Geometry check sheet. Reference: the model listing, model coordinates, mm. A direction names the side the tool comes from. Coordinates: 2 decimals unless noted, no trailing zeros. Write each loop counter-clockwise with the first axis right and the second up, starting at its lowest first coordinate (ties: lowest second). Pieces come first, ordered by that corner, then holes. Notation, with made-up numbers: (44.25, -11) -> (101.25, -11) arc R21 ccw to (101.25, 21) -> close; hole circle Ø2 at (-17.75, -11.75). An arc over 180 degrees is marked (long way). Use a Markdown table: item, result.
```python
from build123d import *

# Parameters (mm, degrees)
F0_R     = 1.397
F1_DEPTH = 3.175


with BuildPart() as f1:
    # F0 (on Front) → F1 (new body)
    with BuildSketch(Plane.XZ):
        Polygon((38.1, 38.735), (38.1, 60.325), (19.05, 60.325), (19.05, 54.476305), (-19.277798, 54.476305), (-19.277798, 60.325), (-38.1, 60.325), (-38.1, -60.325), (-22.7203, -60.325), (-22.7203, -55.5625), (-24.4348, -55.5625), (-24.4348, -52.3875), (-22.7203, -52.3875), (-22.7203, -50.673), (-19.7993, -50.673), (-19.7993, -52.3875), (-18.0848, -52.3875), (-18.0848, -55.5625), (-19.7993, -55.5625), (-19.7993, -60.325), (19.7993, -60.325), (19.7993, -55.5625), (18.0848, -55.5625), (18.0848, -52.3875), (19.7993, -52.3875), (19.7993, -50.673), (22.7203, -50.673), (22.7203, -52.3875), (24.4348, -52.3875), (24.4348, -55.5625), (22.7203, -55.5625), (22.7203, -60.325), (38.1, -60.325), align=None)
        with Locations((-35.56, -43.815)):
            Circle(F0_R, mode=Mode.SUBTRACT)
        with Locations((35.56, -43.815)):
            Circle(F0_R, mode=Mode.SUBTRACT)
        with Locations((-25.4, 27.559)):
            Circle(F0_R, mode=Mode.SUBTRACT)
        with Locations((-35.56, 57.785)):
            Circle(F0_R, mode=Mode.SUBTRACT)
        with Locations((-25.4, 49.911)):
            Circle(F0_R, mode=Mode.SUBTRACT)
        Polygon((-19.05, 24.60625), (19.05, 24.60625), (19.05, 16.51), (24.60625, 16.51), (24.60625, -16.51), (19.05, -16.51), (19.05, -24.60625), (-19.05, -24.60625), (-19.05, -16.51), (-24.60625, -16.51), (-24.60625, 16.51), (-19.05, 16.51), align=None, mode=Mode.SUBTRACT)
        with Locations((25.4, 27.559)):
            Circle(F0_R, mode=Mode.SUBTRACT)
        with Locations((25.4, 49.911)):
            Circle(F0_R, mode=Mode.SUBTRACT)
        with Locations((35.56, 57.785)):
            Circle(F0_R, mode=Mode.SUBTRACT)
    extrude(amount=F1_DEPTH)


solid = f1.part
```
Item 1: Depth check by flat-ended pin: P1, Ø1.5, axis at x = -7, y = -2, coming from the +Z side. Enter the tip coordinate at first touch or a pass-through.
Answer block:
| item | result |
|---|---|
| P1 | stops at z = 54.48 |
Item 2: Tool access check on faces 3 (the flat face through (21, -2, -50.673)), 4 (the flat face through (-29, -2, 60.325)), 5 (the flat face through (0, -2, 24.606)), 6 (the flat face through (19.05, -2, 57)). Record the directions out of +Z, -Z, +X, -X, +Y, -Y that give a thin tool (end or side, any length) a straight path to the whole face; none if there is none.
Answer block:
| item | result |
|---|---|
| face 3 | -Z, +Y, -Y |
| face 4 | +Z, +X, -X, +Y, -Y |
| face 5 | +Y, -Y |
| face 6 | +Z, +Y, -Y |
Item 3: Section check C-C on x = 35.56. Record the boundary of the cut face in (y, z) (3 decimals).
Answer block:
| item | result |
|---|---|
| outline | (-3.175, -60.325) -> (0, -60.325) -> (0, -45.212) -> (-3.175, -45.212) -> close; (-3.175, -42.418) -> (0, -42.418) -> (0, 56.388) -> (-3.175, 56.388) -> close; (-3.175, 59.182) -> (0, 59.182) -> (0, 60.325) -> (-3.175, 60.325) -> close |
Item 4: Thickness scan on L1, parallel to Z at x = 35.56, y = -1.1 (3 decimals); L2, parallel to Z at x = -25.4, y = -1.9 (3 decimals); L3, parallel to X at y = -1.1, z = 17.5. Record the ranges inside material, lowest first. Write a range as [from, to].
Answer block:
| item | result |
|---|---|
| L1 | z = [-60.325, -45.212], [-42.418, 56.388], [59.182, 60.325] |
| L2 | z = [-60.325, 26.162], [28.956, 48.514], [51.308, 60.325] |
| L3 | x = [-38.1, -19.05], [19.05, 38.1] |
Item 5: Section check B-B on z = 5.5. Record the boundary of the cut face in (x, y) (3 decimals).
Answer block:
| item | result |
|---|---|
| outline | (-38.1, -3.175) -> (-24.606, -3.175) -> (-24.606, 0) -> (-38.1, 0) -> close; (24.606, -3.175) -> (38.1, -3.175) -> (38.1, 0) -> (24.606, 0) -> close |
Item 6: Section check A-A on x = 1.5. Record the boundary of the cut face in (y, z) (3 decimals), then the cut area to 3 significant figures.
Answer block:
| item | result |
|---|---|
| outline | (-3.175, -60.325) -> (0, -60.325) -> (0, -24.606) -> (-3.175, -24.606) -> close; (-3.175, 24.606) -> (0, 24.606) -> (0, 54.476) -> (-3.175, 54.476) -> close |
| area | 208 mm^2 |
Item 7: Section check D-D on y = -1.45. Count the separate pieces of the cut face and the enclosed holes in it, then the cut area to 3 significant figures.
Answer block:
| item | result |
|---|---|
| separate pieces | 1 |
| enclosed holes | 9 |
| area | 6,600 mm^2 |
Item 8: Mould release check, pull along X, two halves, no side actions. Record for faces 1 (the flat face through (-22, -2, -16.51)), 2 (the flat face through (0, -2, -60.325)): +X half, -X half, draft (parallel to the pull), parting line (faces both ways), or undercut.
Answer block:
| item | result |
|---|---|
| face 1 | undercut |
| face 2 | draft |
